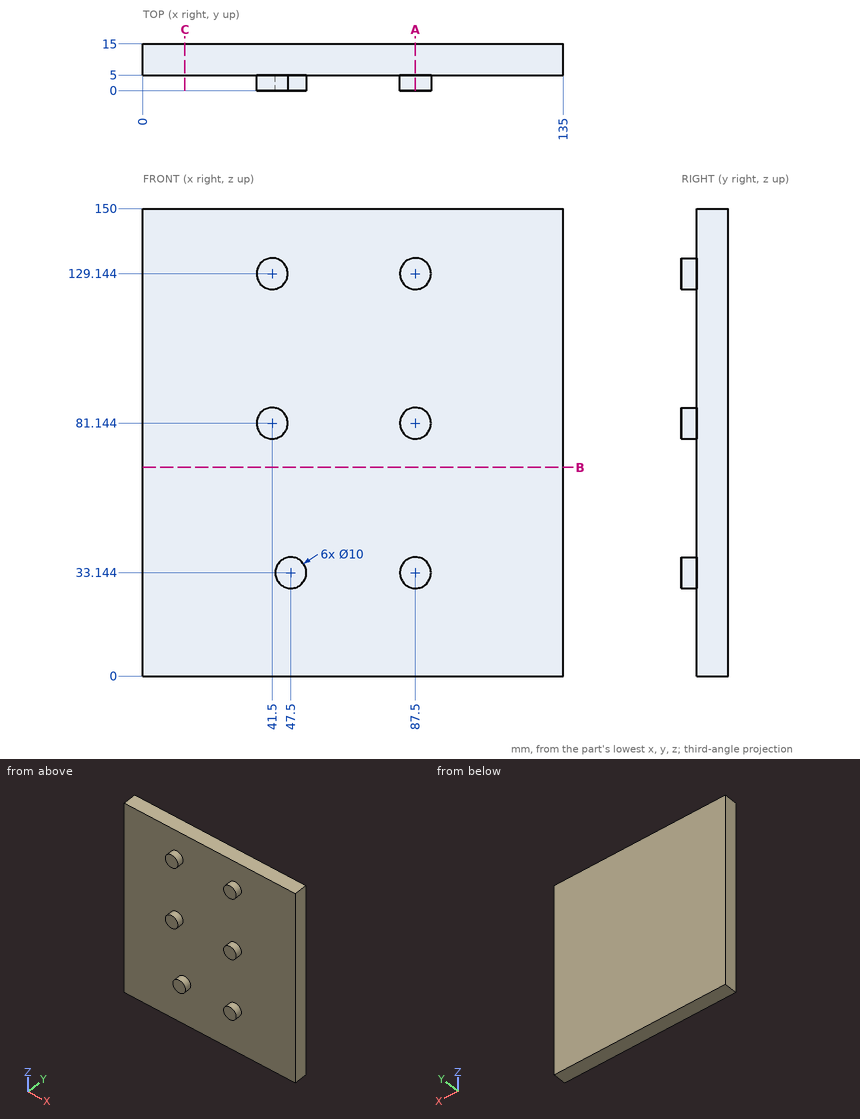
Design review of the part shown in the three views and the two pictorial views. Dimensions are in mm from the part's minimum x, y and z. Coordinates: 2 decimals unless noted, no trailing zeros. Loops run counter-clockwise (first coordinate to the right, second up) from the corner with the lowest first, then second, coordinate; pieces in that order, holes last. Notation, with made-up numbers: M 75.5,-17.5 L 101.5,-17.5 A16 cw 101.5,-4.5 Z; hole C 24,2.5 d3. An arc over 180 degrees is marked long. Put each result on its own line as item: value. Start each with the question number.
Q1. Clearance check with flat-ended pins moving along their axes: pin 1 (2 mm diameter, centred on x = 15.5, z = 112, fed in from -Y); pin 2 (2 mm diameter, centred on x = 117.5, y = 3.5, fed in from +Z). State where each tip first meets the part, or that it passes through.
Q2. Add section B-B (z = 67). Write out the cut boundary in (x, y).
Q3. Add section C-C (x = 13.5). Write out the cut boundary in (y, z).
Q4. Wall thickness on line 1 (Y direction, x = 62, z = 133.5); line 2 (Z direction, x = 45, y = 1.25) (1 decimal): over which ranges is each line inside the solid? List them lowest first.
Q5. Add section A-A (x = 87.5). Write out the cut boundary in (y, z) (1 decimal).
Answers:
1. pin 1: stops at y = 5
1. pin 2: passes through
2. outline: M 0,5 L 135,5 L 135,15 L 0,15 Z
3. outline: M 5,0 L 15,0 L 15,150 L 5,150 Z
4. line 1: y = 5 to 15
4. line 2: z = 28.8 to 37.5, 77.6 to 84.7, 125.6 to 132.7
5. outline: M 0,28.1 L 5,28.1 L 5,0 L 15,0 L 15,150 L 5,150 L 5,134.1 L 0,134.1 L 0,124.1 L 5,124.1 L 5,86.1 L 0,86.1 L 0,76.1 L 5,76.1 L 5,38.1 L 0,38.1 Z
